Part model, mm, in its own coordinate system. Round coordinates to 2 decimals unless told otherwise and drop trailing zeros. Order: outer loops, then holes, each group sorted by start corner. A loop starts at its lowest first (then second) coordinate and runs counter-clockwise, first axis right, second up. Notation, with made-up numbers: M 63,-32.5 L 76,-32.5 A14 ccw 76,-13.5 Z; hole C 69,62.25 d4. An arc over 180 degrees is marked long. Write each question's results on one line, items separated by ' | '. Start each with the question number.
1. Band-saw the part on D-D, the plane z = 2.5. List the corners of the cut face in (x, y).
2. Probe L1, parallel to Z at x = 0, y = -0.4; L2, parallel to X at y = -0.35, z = -0.5; L3, parallel to X at y = -0.3, z = 2.75. List the from-to ranges inside material, lowest first. Write a range as [from, to].
3. Band-saw the part on A-A, the plane x = 0. List the corners of the cut face in (y, z).
4. Band-saw the part on B-B, the plane y = -0.2. List the corners of the cut face in (x, z).
5. Two-plate mould, pull along X, no slides. Class faces 1 (the face through (-9, -0.762, -1)), 2 (the face through (-24.3, -0.4, -4.1)), 3 (the face through (-1.837, -0.376, 0.081)): +X half, -X half, draft (parallel to the pull), parting line (faces both ways), or undercut.
6. Band-saw the part on C-C, the plane z = 0.75. List the corners of the cut face in (x, y), then the cut area to 3 significant figures.
```python
from build123d import *

# Parameters (mm, degrees)
F0_R     = 1.838713
F1_DEPTH = 0.762


with BuildPart() as f1:
    # F0 (on Front) → F1 (new body)
    with BuildSketch(Plane.XZ):
        with BuildLine():
            Line((7.552237, 3.078119), (-22.179499, 3.078119))
            ThreePointArc((-22.179499, 3.078119), (-24.356058, 2.176559), (-25.257618, 0))
            Line((-25.257618, 0), (-25.257618, -2.423407))
            ThreePointArc((-25.257618, -2.423407), (-24.289763, -4.111575), (-22.488076, -4.846813))
            Line((-22.488076, -4.846813), (-22.152904, -4.846813))
            Line((-22.152904, -4.846813), (7.552237, -4.846813))
            Line((7.552237, -4.846813), (7.552237, 3.078119))
        make_face()
        Circle(F0_R, mode=Mode.SUBTRACT)
    extrude(amount=F1_DEPTH)


solid = f1.part
```
Solution:
1) outline: M -23.98,-0.76 L 7.55,-0.76 L 7.55,0 L -23.98,0 Z
2) L1: [-4.85, -1.84], [1.84, 3.08] | L2: [-25.26, -1.77], [1.77, 7.55] | L3: [-23.56, 7.55]
3) outline: M -0.76,-4.85 L 0,-4.85 L 0,-1.84 L -0.76,-1.84 Z; M -0.76,1.84 L 0,1.84 L 0,3.08 L -0.76,3.08 Z
4) outline: M -25.26,-2.42 A2.99 ccw -22.49,-4.85 L 7.55,-4.85 L 7.55,3.08 L -22.18,3.08 A3.08 ccw -25.26,0 Z; hole C 0,0 d3.68
5) face 1: draft | face 2: -X half | face 3: undercut
6) outline: M -25.16,-0.76 L -1.68,-0.76 L -1.68,0 L -25.16,0 Z; M 1.68,-0.76 L 7.55,-0.76 L 7.55,0 L 1.68,0 Z | area: 22.4 mm^2
